```python
from build123d import *

# Parameters (mm, degrees)
SKETCH_1_R      = 40
SKETCH_1_R_2    = 33
EXTRUDE_1_DEPTH = 4
EXTRUDE_START   = 8
SKETCH_2_R      = 40
SKETCH_2_R_2    = 36
EXTRUDE_2_DEPTH = 8
EXTRUDE_3_DEPTH = 3


with BuildPart() as part:
    # 草图1 → 凸台-拉伸1 (new body)
    with BuildSketch(Plane.XY):
        with Locations((-86.606649797, -63.783530386)):
            Circle(SKETCH_1_R)
        with Locations((-86.606649797, -63.783530386)):
            Circle(SKETCH_1_R_2, mode=Mode.SUBTRACT)
    extrude(amount=EXTRUDE_1_DEPTH)

    # 草图2 → 凸台-拉伸2 (add)
    with BuildSketch(Plane(origin=(0, 0, 0), x_dir=(-1, 0, 0), z_dir=(0, 0, -1)).offset(EXTRUDE_START)):
        with Locations((86.606649797, -63.783530386)):
            Circle(SKETCH_2_R)
        with Locations((86.606649797, -63.783530386)):
            Circle(SKETCH_2_R_2, mode=Mode.SUBTRACT)
    extrude(amount=-EXTRUDE_2_DEPTH)

    # 草图4 → 凸台-拉伸3 (add)
    with BuildSketch(Plane.XY.offset(4)):
        with BuildLine():
            Line((-102.470674133, 52.025849932), (-145.802574452, 37.009933401))
            Line((-145.802574452, 37.009933401), (-118.238289751, -42.533185695))
            ThreePointArc((-118.238289751, -42.533185695), (-99.084005703, -27.777233919), (-74.906389432, -27.517269163))
            Line((-74.906389432, -27.517269163), (-102.470674133, 52.025849932))
        make_face()
    extrude(amount=-EXTRUDE_3_DEPTH)


solid = part.part
```
Geometry check sheet. Reference: the model listing, model coordinates, mm. A direction names the side the tool comes from. Round coordinates to 2 decimals unless told otherwise and drop trailing zeros. Loops run counter-clockwise (first coordinate to the right, second up) from the corner with the lowest first, then second, coordinate; pieces in that order, holes last. Notation, with made-up numbers: (-22, 56.5) - (6, 56.5) arc R15 cw to (6, 66.5) - close; hole circle Ø11 at (60, -7). An arc over 180 degrees is marked (long way). Use a Markdown table: item, result.
Q1. Cross-section at B-B on x = -100. Record the cut outline in (y, z).
Solutions:
| item | result |
|---|---|
| outline | (-101.47, -8) - (-97.2, -8) - (-97.2, 0) - (-93.94, 0) - (-93.94, 4) - (-101.47, 4) - close; (-33.62, 0) - (-30.37, 0) - (-30.37, -8) - (-26.09, -8) - (-26.09, 1) - (44.9, 1) - (44.9, 4) - (-33.62, 4) - close |
Q2. Cross-section at D-D on x = -67. Record the cut outline in (y, z), plus the area to 3 significant figures.
Solutions:
| item | result |
|---|---|
| outline | (-98.65, -8) - (-93.98, -8) - (-93.98, 0) - (-90.33, 0) - (-90.33, 4) - (-98.65, 4) - close; (-37.24, 0) - (-33.59, 0) - (-33.59, -8) - (-28.92, -8) - (-28.92, 4) - (-37.24, 4) - close |
| area | 141 mm2 |
Q3. Draft check along Y on faces 4 (the flat face through (-111, 6, 1)), 5 (the flat face through (-57, -80, 0)), 6 (the flat face through (-123.833, 44.623, 2.521)), 7 (the cylindrical face through (-93.76, -96, 1.97)). Enter one of: released by +Y, released by -Y, zero draft, split by the parting line, or undercut.
Solutions:
| item | result |
|---|---|
| face 4 | zero draft |
| face 5 | undercut |
| face 6 | released by +Y |
| face 7 | undercut |
Q4. Material ranges on line 1 (Z direction, x = -86, y = -20); line 2 (Y direction, x = -62, z = -4.25); line 3 (Y direction, x = -114, z = 1.25), recorded low to high.
Solutions:
| item | result |
|---|---|
| line 1 | z = 1 to 4 |
| line 2 | y = -95.32 to -90.06, -37.51 to -32.25 |
| line 3 | y = -92.93 to -82.18, -45.38 to 48.03 |
Q5. Go/stop test with flat-tipped pins: P1, Ø6, axis at x = -65.5, z = -3.5, coming from the +Y side; P2, Ø4, axis at y = -30, z = 1, coming from the +X side; P3, Ø10, axis at x = -92, y = 2, coming from the -Z side. Record where each tip stops, or that it passes through.
Solutions:
| item | result |
|---|---|
| P1 | stops at y = -28.12 |
| P2 | stops at x = -62.32 |
| P3 | stops at z = 1 |
Q6. Cross-section at A-A on y = -59.5. Record the cut outline in (x, z), plus the area to 3 significant figures.
Solutions:
| item | result |
|---|---|
| outline | (-126.38, -8) - (-122.35, -8) - (-122.35, 0) - (-119.33, 0) - (-119.33, 4) - (-126.38, 4) - close; (-53.89, 0) - (-50.86, 0) - (-50.86, -8) - (-46.84, -8) - (-46.84, 4) - (-53.89, 4) - close |
| area | 121 mm2 |
Q7. Access from +Z, -Z, +X, -X, +Y, -Y to the whole of each face (thin tool, end or side, straight path). Record for faces 1 (the flat face through (-132.59, -1.12, 2.52)), 2 (the cylindrical face through (-58.04, -85.69, -4.06)), 3 (the flat face through (-88.884, 12.818, 2.521)).
Solutions:
| item | result |
|---|---|
| face 1 | +Z, -Z, -X |
| face 2 | -Z |
| face 3 | +Z, -Z, +X, +Y |
Q8. Cross-section at C-C on z = -4.25. Record the cut outline in (x, y).
Solutions:
| item | result |
|---|---|
| outline | circle Ø80 at (-86.61, -63.78); hole circle Ø72 at (-86.61, -63.78) |
